Input: part model. Units: mm. Frame: model coordinates. A direction names the side the tool comes from. Give positions to 0.01 mm unless a question says otherwise; leave off trailing zeros. Order: outer loops, then holes, each group sorted by start corner. A loop starts at its lowest first (then second) coordinate and runs counter-clockwise, first axis right, second up. Notation, with made-up numbers: (55.25, 42) - (75.25, 42) arc R25 ccw to (75.25, 71) - close; hole circle Ø5 at (-2.75, 2.25). An arc over 180 degrees is marked (long way). Answer in a Markdown table with one row per item. Add a question column.
from build123d import *

# Parameters (mm, degrees)
CROQUIS1_W              = 240
CROQUIS1_H              = 60
CROQUIS1_R              = 14
SALIENTE_EXTRUIR1_DEPTH = 3
CROQUIS4_W              = 90
CROQUIS4_H              = 60
CORTAR_EXTRUIR2_DEPTH   = 5
CROQUIS2_W              = 150
CROQUIS2_H              = 60
CROQUIS2_W_2            = 144
CROQUIS2_H_2            = 54
SALIENTE_EXTRUIR2_DEPTH = 195
CROQUIS5_R              = 11
CORTAR_EXTRUIR3_DEPTH   = 5


with BuildPart() as part:
    # Croquis1 → Saliente-Extruir1 (new body)
    with BuildSketch(Plane(origin=(0, 0, 0), x_dir=(1, 0, 0), z_dir=(0, 1, 0))):
        Rectangle(CROQUIS1_W, CROQUIS1_H)
        Circle(CROQUIS1_R, mode=Mode.SUBTRACT)
        with Locations((-90, 0)):
            Circle(CROQUIS1_R, mode=Mode.SUBTRACT)
    extrude(amount=SALIENTE_EXTRUIR1_DEPTH)

    # Croquis4 → Cortar-Extruir2 (cut)
    with BuildSketch(Plane(origin=(0, 3, 0), x_dir=(1, 0, 0), z_dir=(0, 1, 0))):
        with Locations((75, 0)):
            Rectangle(CROQUIS4_W, CROQUIS4_H)
    extrude(amount=-CORTAR_EXTRUIR2_DEPTH, mode=Mode.SUBTRACT)

    # Croquis2 → Saliente-Extruir2 (add)
    with BuildSketch(Plane.XZ):
        with Locations((-45, 0)):
            Rectangle(CROQUIS2_W, CROQUIS2_H)
        with Locations((-45, 0)):
            Rectangle(CROQUIS2_W_2, CROQUIS2_H_2, mode=Mode.SUBTRACT)
    extrude(amount=SALIENTE_EXTRUIR2_DEPTH)

    # Croquis5 → Cortar-Extruir3 (cut)
    with BuildSketch(Plane.XY.offset(30)):
        with Locations((-45, -90)):
            Circle(CROQUIS5_R)
    extrude(amount=-CORTAR_EXTRUIR3_DEPTH, mode=Mode.SUBTRACT)


solid = part.part
Q1. Line query: probe 1 along X at (y, z) = (1.6, 0); probe 2 along X at (y, z) = (-53, 9); probe 3 along Z at (x, y) = (-47.5, -139.5). Output: solid intervals per line, ascending.
Q2. Section C-C, the plane y = -128.5. Return loops of the section in (x, z), then the cut area to 3 significant figures.
Q3. Section A-A, the plane x = 0. Return loops of the section in (y, z).
Q4. Section D-D, the plane x = -111. Return loops of the section in (y, z), then the cut area to 3 significant figures.
Q5. Section B-B, the plane z = 0. Return loops of the section in (x, y).
Q6. Access query for faces 1 (the flat face through (-46, 3, 0)), 2 (the flat face through (-46, 0, 0)), 3 (the cylindrical face through (-46.432, -79.094, 28.521)). Directions: +Z, -Z, +X, -X, +Y, -Y. A direction counts if a zero-diameter tool reaches every point of the face in a straight line with its end or side. Return the directions, or none.
Q7. Pull-direction query (X, two-part tool) for faces 4 (the flat face through (-68, -195, 29)), 5 (the flat face through (-120, -95, 0)), 6 (the flat face through (-117, -96, 0)); classes: +X half, -X half, draft (parallel to the pull), parting line (faces both ways), or undercut.
Computed:
| question | item | result |
|---|---|---|
| 1 | probe 1 | x = -120 to -104, -76 to -14, 14 to 30 |
| 1 | probe 2 | x = -120 to -117, 27 to 30 |
| 1 | probe 3 | z = -30 to -27, 27 to 30 |
| 2 | outline | (-120, -30) - (30, -30) - (30, 30) - (-120, 30) - close; hole (-117, -27) - (27, -27) - (27, 27) - (-117, 27) - close |
| 2 | area | 1,220 mm^2 |
| 3 | outline | (-195, -30) - (3, -30) - (3, -14) - (0, -14) - (0, -27) - (-195, -27) - close; (-195, 27) - (0, 27) - (0, 14) - (3, 14) - (3, 30) - (-195, 30) - close |
| 4 | outline | (-195, -30) - (3, -30) - (3, 30) - (-195, 30) - (-195, 27) - (0, 27) - (0, -27) - (-195, -27) - close |
| 4 | area | 1,350 mm^2 |
| 5 | outline | (-120, -195) - (-117, -195) - (-117, 0) - (-104, 0) - (-104, 3) - (-120, 3) - close; (-76, 0) - (-14, 0) - (-14, 3) - (-76, 3) - close; (14, 0) - (27, 0) - (27, -195) - (30, -195) - (30, 3) - (14, 3) - close |
| 6 | face 1 | +Z, -Z, +X, -X, +Y |
| 6 | face 2 | -Y |
| 6 | face 3 | +Z |
| 7 | face 4 | draft |
| 7 | face 5 | -X half |
| 7 | face 6 | undercut |
